Verification items for the finished model (mm, model axes). Face numbers are marked on the shaded views. A direction names the side the tool comes from. Round coordinates to 2 decimals unless told otherwise and drop trailing zeros. Write each loop counter-clockwise with the first axis right and the second up, starting at its lowest first coordinate (ties: lowest second). Pieces come first, ordered by that corner, then holes. Notation, with made-up numbers: (-8, 81.5) -> (30, 81.5) arc R10 cw to (30, 95.5) -> close; hole circle Ø2 at (-1.75, -40). An arc over 180 degrees is marked (long way). Answer as a JSON object with one key per item and string values. Group by question number.
(1) Sectioned sample at C-C on z = 0.5. Count the separate pieces of the cut face and the enclosed holes in it, and give its area (3 significant figures).
(2) Draft check along X on the marked faces 1, 2, 3 and 4. Enter one of: released by +X, released by -X, zero draft, split by the parting line, or undercut.
(3) Sectioned sample at B-B on x = 0. Record the cut outline in (y, z) (3 decimals).
(4) Gauge pin test, flat ends, axial feed: pin 1 Ø4 at (x, y) = (-1.5, -8) entering from +Z; pin 2 Ø0.6 at (y, z) = (17, 3) entering from +X; pin 3 Ø1.1 at (x, y) = (3, 15) entering from -Z. Record the tip position at first contact, or that the pin passes through.
(5) Scan lines: L1, parallel to Y at x = 0, z = 0.5 (3 decimals); L2, parallel to Y at x = -1, z = 0.9 (3 decimals); L3, parallel to X at y = -14.05, z = 1.2. Record each from-to range of solid material in increasing order. Write a range as from..to.
(6) Set-up check for the marked faces 5, 6 and 7: record each of +Z, -Z, +X, -X, +Y, -Y from which the full face is reachable in a straight line by a thin tool's end or side.
(7) Sectioned sample at D-D on y = -7. Record the cut outline in (x, z), and give its area (3 significant figures).
(8) Sectioned sample at A-A on y = -3.05. Record the cut outline in (x, z), and give its area (3 significant figures).
Autodesk Inventor part; units mm, degrees
ref_plane "YZ Plane" through (0, 0, 0) normal (1, 0, 0) x (0, 1, 0)
ref_plane "XZ Plane" through (0, 0, 0) normal (0, 1, 0) x (-1, 0, 0)
ref_plane "XY Plane" through (0, 0, 0) normal (0, 0, 1) x (1, 0, 0)
sketch "Sketch1" plane through (0, 0, 0) normal (0, 0, 1) x (1, 0, 0)
  line L0 (0, 26.67) -> (0, -26.67)
  line L1 (-5.7785, 0) -> (5.7785, 0)
  line L2 (4.1275, -19.05) -> (-4.1275, -19.05)
  line L3 (-4.1275, -19.05) -> (-4.1275, 19.05)
  line L4 (-4.1275, 19.05) -> (4.1275, 19.05)
  line L5 (4.1275, 19.05) -> (4.1275, -19.05)
  line L6 (4.1275, -19.05) -> (-4.1275, 19.05) construction
  line L7 (-4.1275, -19.05) -> (4.1275, 19.05) construction
  point P0 (0, 0)
  point P1 (0, -14.05)
  point P2 (0, -3.05)
  dimension "d0" = 38.1
  dimension "d1" = 8.255
  dimension "d2" = 5
  dimension "d3" = 11
extrude "Extrusion1" add sketch "Sketch1" along normal blind 3.81
sketch "Sketch5" plane through (0, 0, 3.81) normal (0, 0, 1) x (1, 0, 0)
  point P0 (0, 0)
  point P1 (0, -3.05)
  point P2 (0, -14.05)
hole "Hole2" at (0, -3.05, 3.81) at (0, -14.05, 3.81) direction (0, 0, -1) diameter 1.27 end through all
sketch "Sketch2" plane through (0, 0, 0) normal (0, 0, -1) x (-1, 0, 0)
  line L0 (4.1275, 19.05) -> (-4.1275, 19.05)
  line L1 (-3.8354, 19.05) -> (-3.8354, 14.0205)
  line L2 (-3.8354, 14.0205) -> (-2.413, 12.827)
  line L3 (-2.413, 12.827) -> (2.413, 12.827)
  line L4 (2.413, 12.827) -> (3.8354, 14.0205)
  line L5 (3.8354, 14.0205) -> (3.8354, 19.05)
  line L6 (0, -26.67) -> (0, 26.67)
  line L7 (-6.6675, 0) -> (6.6675, 0)
  point P0 (0, 0)
  dimension "d13" = 7.6708
  dimension "d14" = 6.223
  dimension "d15" = 4.826
  dimension "d16" = 3.8354
  dimension "d17" = 2.413
  dimension "d18" = 140
extrude "Extrusion2" cut sketch "Sketch2" against normal blind 2.54
sketch "Sketch3" plane through (0, 0, 0) normal (0, 0, -1) x (-1, 0, 0)
  line L0 (-3.8354, 19.05) -> (3.8354, 19.05)
  line L1 (-3.8354, 14.0205) -> (-3.8354, 19.05)
  line L2 (-2.413, 12.827) -> (-3.8354, 14.0205)
  line L3 (2.413, 12.827) -> (-2.413, 12.827)
  line L4 (3.8354, 14.0205) -> (2.413, 12.827)
  line L5 (3.8354, 19.05) -> (3.8354, 14.0205)
  line L6 (0, -26.67) -> (0, 26.67)
  line L7 (2.8575, 14.605) -> (-2.8575, 14.605)
  line L8 (-2.8575, 14.605) -> (-2.8575, 19.05)
  line L9 (-2.8575, 19.05) -> (2.8575, 19.05)
  line L10 (2.8575, 19.05) -> (2.8575, 14.605)
  line L11 (2.8575, 14.605) -> (-2.8575, 19.05) construction
  line L12 (-2.8575, 14.605) -> (2.8575, 19.05) construction
  line L13 (2.413, 5.715) -> (-2.413, 5.715)
  line L14 (-2.413, 5.715) -> (-2.413, 14.605)
  line L15 (-2.413, 14.605) -> (2.413, 14.605)
  line L16 (2.413, 14.605) -> (2.413, 5.715)
  line L17 (2.413, 5.715) -> (-2.413, 14.605) construction
  line L18 (-2.413, 5.715) -> (2.413, 14.605) construction
  point P0 (0, 0)
  point P1 (0, 16.8275)
  point P2 (0, 10.16)
  dimension "d21" = 5.715
  dimension "d22" = 4.826
  dimension "d23" = 8.89
  dimension "d24" = 4.445
extrude "Extrusion3" cut sketch "Sketch3" against normal through all contours L0 L6 L7 L8 | L0 L10 L7 L6 | L14 L7 L6 L3 | L3 L6 L13 L14 | L7 L16 L3 L6 | L3 L16 L13 L6
fillet "Fillet1" radius 0.7937 4 edges at (3.8354, 14.0205, 1.27) (2.413, 12.827, 1.27) (-2.413, 12.827, 1.27) (-3.8354, 14.0205, 1.27)
fillet "Fillet2" radius 0.7937 2 edges at (-2.8575, 14.605, 3.175) (2.8575, 14.605, 3.175)
sketch "Sketch6" plane through (0, 0, 0) normal (0, 0, -1) x (-1, 0, 0)
  line L0 (0, -26.67) -> (0, 26.67)
  line L1 (-8.89, 0) -> (8.89, 0)
  line L2 (6.35, 5.715) -> (-6.35, 5.715)
  line L3 (-6.35, 5.715) -> (-6.35, 19.05)
  line L4 (-6.35, 19.05) -> (6.35, 19.05)
  line L5 (6.35, 19.05) -> (6.35, 5.715)
  line L6 (6.35, 5.715) -> (-6.35, 19.05) construction
  line L7 (-6.35, 5.715) -> (6.35, 19.05) construction
  line L8 (-3.8354, 19.05) -> (-4.1275, 19.05)
  point P0 (0, 0)
  point P1 (0, 12.3825)
  dimension "d50" = 12.7
  dimension "d51" = 5.715
  dimension "d52" = 0
extrude "Extrusion5" cut sketch "Sketch6" against normal blind 1.27
chamfer "Chamfer1" distance 1.27 angle 45 2 edges at (3.9815, 19.05, 1.27) (-3.9814, 19.05, 1.27)
chamfer "Chamfer2" distance 1.016 angle 45 2 edges at (3.4925, 19.05, 3.81) (-3.4925, 19.05, 3.81)
sketch "Sketch7" plane through (0, 0, 3.81) normal (0, 0, 1) x (1, 0, 0)
  line L0 (-4.1275, 18.034) -> (-2.8575, 18.034)
  line L1 (-4.1275, 18.034) -> (-4.1275, -19.05)
  line L2 (-4.1275, -19.05) -> (4.1275, -19.05)
  line L3 (4.1275, -19.05) -> (4.1275, 18.034)
  line L4 (2.8575, 18.034) -> (4.1275, 18.034)
  line L5 (2.8575, 18.034) -> (2.8575, 15.3178)
  arc A0 (2.413, 14.605) -> (2.8575, 15.3178) centre (2.0638, 15.3178) ccw
  line L6 (2.413, 14.605) -> (2.413, 5.715)
  line L7 (2.413, 5.715) -> (-2.413, 5.715)
  line L8 (-2.413, 5.715) -> (-2.413, 14.605)
  arc A1 (-2.8575, 15.3178) -> (-2.413, 14.605) centre (-2.0637, 15.3178) ccw
  line L9 (-2.8575, 15.3178) -> (-2.8575, 18.034)
  circle A2 centre (0, -3.05) radius 0.635
  circle A3 centre (0, -14.05) radius 0.635
  line L10 (-4.1275, -19.05) -> (4.1275, -19.05)
  line L11 (4.1275, -19.05) -> (4.1275, 0)
  line L12 (4.1275, 0) -> (-4.1275, 0)
  line L13 (-4.1275, 0) -> (-4.1275, -19.05)
  line L14 (-6.6675, 0) -> (6.6675, 0)
  line L15 (0, 26.67) -> (0, -26.67)
  line L16 (2.413, 0) -> (-2.413, 0)
  line L17 (-2.413, 0) -> (-2.413, 5.715)
  line L18 (-2.413, 5.715) -> (2.413, 5.715)
  line L19 (2.413, 5.715) -> (2.413, 0)
  line L20 (2.413, 0) -> (-2.413, 5.715) construction
  line L21 (-2.413, 0) -> (2.413, 5.715) construction
  point P0 (0, 0)
  point P1 (0, 2.8575)
  dimension "d55" = 0
  dimension "d58" = 0
extrude "Extrusion6" cut sketch "Sketch7" against normal blind 1.27 contours L12 L15 A2 A3 L2 L1 | L15 A3 A2 L12 L3 L2
hole "Hole3" at (0, -3.05, 2.54) direction (0, 0, -1) diameter 2.3876 end through all countersink diameter 4.3942 countersink angle 90
hole "Hole4" at (0, -14.05, 2.54) direction (0, 0, -1) diameter 2.3876 end through all countersink diameter 4.3942 countersink angle 90
extrude "Extrusion7" cut sketch "Sketch7" against normal up to surface (1.27 mm away) contours L17 L7 L15 L12 | L15 L7 L19 L12
fillet "Fillet3" radius 1.5875 2 edges at (2.413, 5.715, 1.905) (-2.413, 5.715, 1.905)
chamfer "Chamfer4" distance 1.27 angle 45 2 edges at (-4.1275, 9.017, 3.81) (4.1275, 9.017, 3.81)
equation "\"d16\" = 0.5 * d13"
equation "\"d17\" = 0.5 * d15"
properties part number "J007803" material "VERO BLACK"
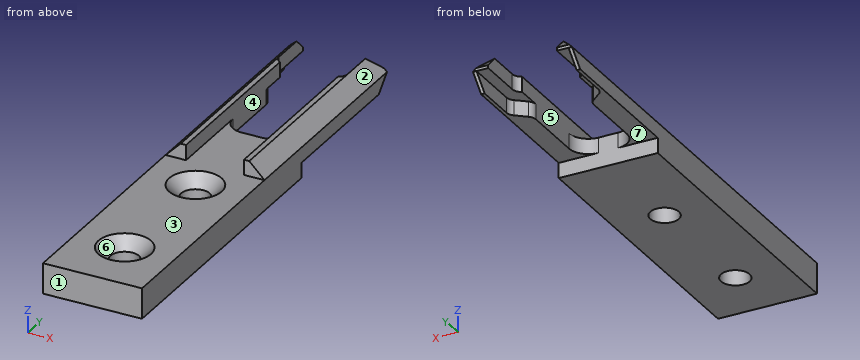
Computed values:
{
 "1": {"separate pieces": "1", "enclosed holes": "2", "area": "195 mm2"},
 "2": {"face 1": "zero draft", "face 2": "released by +X", "face 3": "undercut", "face 4": "undercut"},
 "3": {"outline": "(-19.05, 0) -> (-15.244, 0) -> (-15.244, 1.537) -> (-16.247, 2.54) -> (-19.05, 2.54) -> close; (-12.856, 0) -> (-4.244, 0) -> (-4.244, 1.537) -> (-5.247, 2.54) -> (-11.853, 2.54) -> (-12.856, 1.537) -> close; (-1.856, 0) -> (5.715, 0) -> (5.715, 2.54) -> (-0.853, 2.54) -> (-1.856, 1.537) -> close"},
 "4": {"pin 1": "z = 2.54", "pin 2": "x = 3.97", "pin 3": "z = 2.54"},
 "5": {"L1": "-19.05..-15.244, -12.856..-4.244, -1.856..5.715", "L2": "-19.05..-14.702, -13.398..-3.702, -2.398..5.715", "L3": "-4.13..-1.19, 1.19..4.13"},
 "6": {"face 5": "+Z, +Y", "face 6": "+Z", "face 7": "-Z, +X, -X, +Y"},
 "7": {"outline": "(-4.13, 0) -> (4.13, 0) -> (4.13, 2.54) -> (-4.13, 2.54) -> close", "area": "21.0 mm2"},
 "8": {"outline": "(-4.13, 0) -> (-1.19, 0) -> (-1.19, 1.54) -> (-2.2, 2.54) -> (-4.13, 2.54) -> close; (1.19, 0) -> (4.13, 0) -> (4.13, 2.54) -> (2.2, 2.54) -> (1.19, 1.54) -> close", "area": "13.9 mm2"}
}
